```python
from build123d import *

# Parameters (mm, degrees)
F0_R     = 14
F0_R_2   = 9
F1_DEPTH = 18
F2_R     = 15
F3_DEPTH = 10
F4_R     = 12.75
F4_R_2   = 10.5
F5_DEPTH = 5
F6_R     = 6
F6_R_2   = 3
F7_DEPTH = 5
F8_R     = 12
F8_R_2   = 9
F9_DEPTH = 5


with BuildPart() as f1:
    # F0 (on Top) → F1 (new body)
    with BuildSketch(Plane.XY):
        Circle(F0_R)
        Circle(F0_R_2, mode=Mode.SUBTRACT)
    extrude(amount=F1_DEPTH)

    # F2 (on face) → F3 (join)
    with BuildSketch(Plane(origin=(0, 0, 0), x_dir=(1, 0, 0), z_dir=(0, 0, -1))):
        Circle(F2_R)
    extrude(amount=-F3_DEPTH)

    # F4 (on face) → F5 (cut)
    with BuildSketch(Plane.XY.offset(18)):
        Circle(F4_R)
        Circle(F4_R_2, mode=Mode.SUBTRACT)
    extrude(amount=-F5_DEPTH, mode=Mode.SUBTRACT)

    # F6 (on face) → F7 (cut)
    with BuildSketch(Plane(origin=(0, 0, 0), x_dir=(1, 0, 0), z_dir=(0, 0, -1))):
        Circle(F6_R)
        Circle(F6_R_2, mode=Mode.SUBTRACT)
    extrude(amount=-F7_DEPTH, mode=Mode.SUBTRACT)

    # F8 (on face) → F9 (cut)
    with BuildSketch(Plane(origin=(0, 0, 0), x_dir=(1, 0, 0), z_dir=(0, 0, -1))):
        Circle(F8_R)
        Circle(F8_R_2, mode=Mode.SUBTRACT)
    extrude(amount=-F9_DEPTH, mode=Mode.SUBTRACT)


solid = f1.part
```
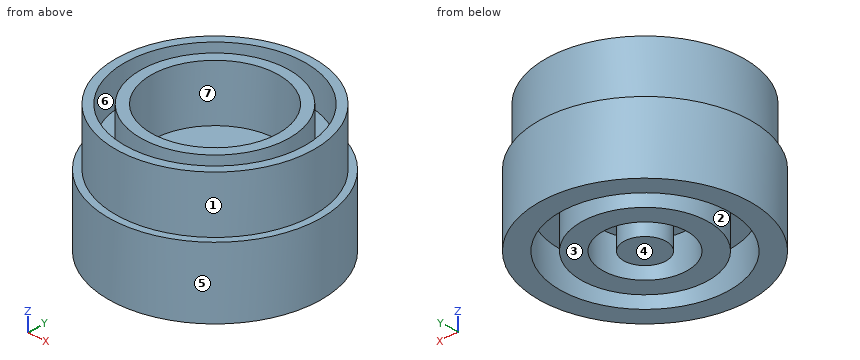
Can you work these out from the model? Positions are in its coordinate system, mm. Face numbers are marked on the shaded views. A direction names the side the tool comes from. Coordinates: 2 decimals unless noted, no trailing zeros. Loops run counter-clockwise (first coordinate to the right, second up) from the corner with the lowest first, then second, coordinate; pieces in that order, holes last.
1) Imagine slicing it at B-B on z = 14. List the corners of the cut face in (x, y) for me, plus the area to 3 significant figures.
2) I need wall thicknesses on probe 1 along Y at (x, z) = (0, 15.95); probe 2 along X at (y, z) = (0, 1.65). Which ranges of each line are inside material? Lowest first, please.
3) Imagine slicing it at D-D on x = 7.75. List the corners of the cut face in (y, z) for me, plus the area to 3 significant figures.
4) Thinking about a two-plate mould opening in X: for the marked faces 4, 5, 6 and 7, which applies, pulls with the +X half, pulls with the -X half, needs draft (parallel to the pull), parting line crosses it, or undercut?
5) For pin 1 (6 mm diameter, centred on x = 5, z = 7.5, fed in from -Y); pin 2 (1 mm diameter, centred on x = 11.5, z = 11.5, fed in from +Y); pin 3 (2 mm diameter, centred on y = 5.5, z = 4.5, fed in from +X), each with a flat end and sliding along its axis, tell me the tip position at first contact or that it passes through.
6) Which directions (+Z, -Z, +X, -X, +Y, -Y) give clear straight access to the entire face, cutting with the end or side of a thin tool? Please do the marked faces 1, 2 and 3.
7) Imagine slicing it at A-A on z = 3.75. List the corners of the cut face in (x, y) for me.
8) Imagine slicing it at C-C on y = -7. List the corners of the cut face in (x, z) for me, plus the area to 3 significant figures.
Completed:
1. outline: circle Ø28 at (0, 0); circle Ø21 at (0, 0); hole circle Ø25.5 at (0, 0); hole circle Ø18 at (0, 0)
1. area: 197 mm2
2. probe 1: y = -14 to -12.75, -10.5 to -9, 9 to 10.5, 12.75 to 14
2. probe 2: x = -15 to -12, -9 to -6, -3 to 3, 6 to 9, 12 to 15
3. outline: (-12.84, 0) - (-9.16, 0) - (-9.16, 5) - (-4.58, 5) - (-4.58, 0) - (4.58, 0) - (4.58, 5) - (9.16, 5) - (9.16, 0) - (12.84, 0) - (12.84, 10) - (11.66, 10) - (11.66, 18) - (10.12, 18) - (10.12, 13) - (7.08, 13) - (7.08, 18) - (4.58, 18) - (4.58, 10) - (-4.58, 10) - (-4.58, 18) - (-7.08, 18) - (-7.08, 13) - (-10.12, 13) - (-10.12, 18) - (-11.66, 18) - (-11.66, 10) - (-12.84, 10) - close
3. area: 294 mm2
4. face 4: needs draft
4. face 5: parting line crosses it
4. face 6: undercut
4. face 7: undercut
5. pin 1: stops at y = -14.87
5. pin 2: stops at y = 8.66
5. pin 3: stops at x = 14.31
6. face 1: +Z
6. face 2: -Z
6. face 3: -Z, +X, -X, +Y, -Y
7. outline: circle Ø30 at (0, 0); circle Ø18 at (0, 0); circle Ø6 at (0, 0); hole circle Ø24 at (0, 0); hole circle Ø12 at (0, 0)
8. outline: (-13.27, 0) - (-9.75, 0) - (-9.75, 5) - (-5.66, 5) - (-5.66, 0) - (5.66, 0) - (5.66, 5) - (9.75, 5) - (9.75, 0) - (13.27, 0) - (13.27, 10) - (12.12, 10) - (12.12, 18) - (10.66, 18) - (10.66, 13) - (7.83, 13) - (7.83, 18) - (5.66, 18) - (5.66, 10) - (-5.66, 10) - (-5.66, 18) - (-7.83, 18) - (-7.83, 13) - (-10.66, 13) - (-10.66, 18) - (-12.12, 18) - (-12.12, 10) - (-13.27, 10) - close
8. area: 300 mm2
